from build123d import *

# Parameters (mm, degrees)
ESQUISSE1_R             = 16
BOSS_EXTRU_1_DEPTH      = 36.4
ESQUISSE2_R             = 9.5
BOSS_EXTRU_2_DEPTH      = 2.25
ESQUISSE3_R             = 5
BOSS_EXTRU_3_DEPTH      = 2.6
ESQUISSE4_R             = 3
BOSS_EXTRU_4_DEPTH      = 16
CONG_1_R                = 0.25
ESQUISSE6_R             = 1.3
ENL_V_MAT_EXTRU_1_DEPTH = 7
ESQUISSE7_R             = 2
ENL_V_MAT_EXTRU_2_DEPTH = 13.8


with BuildPart() as part:
    # Esquisse1 → Boss.-Extru.1 (new body)
    with BuildSketch(Plane.XY):
        Circle(ESQUISSE1_R)
    extrude(amount=BOSS_EXTRU_1_DEPTH)

    # Esquisse2 → Boss.-Extru.2 (add)
    with BuildSketch(Plane.XY.offset(36.4)):
        Circle(ESQUISSE2_R)
    extrude(amount=BOSS_EXTRU_2_DEPTH)

    # Esquisse3 → Boss.-Extru.3 (add)
    with BuildSketch(Plane.XY.offset(38.65)):
        Circle(ESQUISSE3_R)
    extrude(amount=BOSS_EXTRU_3_DEPTH)

    # Esquisse4 → Boss.-Extru.4 (add)
    with BuildSketch(Plane.XY.offset(41.25)):
        Circle(ESQUISSE4_R)
    extrude(amount=BOSS_EXTRU_4_DEPTH)

    # Congé1
    cong_1_edges = [part.edges().sort_by_distance(p)[0] for p in [
        (-5, 0, 41.25),
        (-3, 0, 57.25),
        (-16, 0, 36.4),
        (-9.5, 0, 38.65),
    ]]
    fillet(cong_1_edges, radius=CONG_1_R)

    # Esquisse6 → Enlèv. mat.-Extru.1 (cut)
    with BuildSketch(Plane.XY.offset(36.4)):
        with Locations((0, 13)):
            Circle(ESQUISSE6_R)
        with Locations((-13, 0)):
            Circle(ESQUISSE6_R)
        with Locations((13, 0)):
            Circle(ESQUISSE6_R)
        with Locations((0, -13)):
            Circle(ESQUISSE6_R)
    extrude(amount=-ENL_V_MAT_EXTRU_1_DEPTH, mode=Mode.SUBTRACT)

    # Esquisse7 → Enlèv. mat.-Extru.2 (cut)
    with BuildSketch(Plane(origin=(0, 0, 0), x_dir=(-1, 0, 0), z_dir=(0, 0, -1))):
        Circle(ESQUISSE7_R)
    extrude(amount=-ENL_V_MAT_EXTRU_2_DEPTH, mode=Mode.SUBTRACT)


solid = part.part
Source: CAD feature listing. Evaluate the final solid. Frame: model axes, mm. A direction names the side the tool comes from. Round coordinates to 2 decimals unless told otherwise and drop trailing zeros. Loops run counter-clockwise (first coordinate to the right, second up) from the corner with the lowest first, then second, coordinate; pieces in that order, holes last. Notation, with made-up numbers: M 78,23.25 L 98,23.25 A19 cw 98,29.25 Z; hole C 25.25,87.5 d11. An arc over 180 degrees is marked long. Answer as CSV lines item,"result".
Q1. Cut plane A-A (z = 31.5). Return the cut outline in (x, y), plus the area to 3 significant figures.
Verdict:
outline,"C 0,0 d32; hole C -13,0 d2.6; hole C 0,-13 d2.6; hole C 0,13 d2.6; hole C 13,0 d2.6"
area,"783 mm^2"
Q2. Cut plane C-C (z = 18). Return the cut outline in (x, y).
Verdict:
outline,"C 0,0 d32"
Q3. Line query: line 1 along Y through (x, z) = (0, 34.25); line 2 along Z through (x, y) = (7.5, -2); line 3 along Z through (x, y) = (1, 4.5). Output: solid intervals per line, ascending.
Verdict:
line 1,"y = -16 to -14.3, -11.7 to 11.7, 14.3 to 16"
line 2,"z = 0 to 38.65"
line 3,"z = 0 to 41.25"
Q4. Reachability of faces 5 (the face through (0, -2, 7)), 6 (the face through (-11.76, 0.39, 32.95)), 7 (the face through (0, 0, 57.25)) from +Z, -Z, +X, -X, +Y, -Y: full face, straight path, thin tool, end or side. Return the list, or none.
Verdict:
face 5,"-Z"
face 6,"+Z"
face 7,"+Z, +X, -X, +Y, -Y"
Q5. Pull-direction query (Y, two-part tool) for faces 1 (the face through (13, 0, 29.4)), 2 (the face through (-3, 0, 49)), 3 (the face through (0, 0, 13.8)), 4 (the face through (3, 0, 0)); classes: +Y half, -Y half, draft (parallel to the pull), parting line (faces both ways), or undercut.
Verdict:
face 1,"undercut"
face 2,"parting line"
face 3,"undercut"
face 4,"draft"
Q6. Cut plane B-B (z = 53). Return the cut outline in (x, y).
Verdict:
outline,"C 0,0 d6"
Q7. Contact query for flat-ended pins moving along their axis: pin 1 (1.3 mm diameter, centred on x = 0, y = 13, fed in from +Z); pin 2 (1.5 mm diameter, centred on x = -8, y = 5, fed in from +Z); pin 3 (2 mm diameter, centred on x = -8.5, y = -8.5, fed in from +Z). Output: stop coordinate, or through.
Verdict:
pin 1,"stops at z = 29.4"
pin 2,"stops at z = 38.65"
pin 3,"stops at z = 36.4"
